```python
from build123d import *

# Parameters (mm, degrees)
BOSS_EXTRUDE1_DEPTH = 8.255
FILLET1_R           = 4.191
SKETCH2_R           = 2.07899
CUT_EXTRUDE1_DEPTH  = 81.896006892
FILLET2_R           = 4.191
SKETCH3_R           = 2.07899
CUT_EXTRUDE2_DEPTH  = 8.255


with BuildPart() as part:
    # Sketch1 → Boss-Extrude1 (new body)
    with BuildSketch(Plane(origin=(0, 0, 0), x_dir=(1, 0, 0), z_dir=(0, 1, 0))):
        Polygon((69.85, -7.99998), (69.85, -9.99998), (0, -9.99998), (0, -8.001), (9.99998, -8.001), (9.99998, -1.99898), (0, -1.99898), (0, 0), (69.85, 0), (69.85, -2), (79.84998, -2), (79.84998, -7.99998), align=None)
    extrude(amount=BOSS_EXTRUDE1_DEPTH)

    # Fillet1
    # the kernel refuses this fillet: 4.191 mm, written as the material it takes off along each edge
    with BuildSketch(Plane(origin=(0, 0, 12.47648), x_dir=(0, 1, 0), z_dir=(0, 0, -1)), Plane(origin=(0, 0, 20.47748), x_dir=(0, 1, 0), z_dir=(0, 0, -1))) as fillet1_piece_1:
        with BuildLine():
            CenterArc((FILLET1_R, FILLET1_R), FILLET1_R, 180, 90)
            Line((0, FILLET1_R), (0, 0))
            Line((0, 0), (FILLET1_R, 0))
        make_face()
    extrude(amount=22.95398, mode=Mode.SUBTRACT)
    with BuildSketch(Plane(origin=(0, 8.255, 12.47648), x_dir=(0, -1, 0), z_dir=(0, 0, -1)), Plane(origin=(0, 8.255, 20.47748), x_dir=(0, -1, 0), z_dir=(0, 0, -1))) as fillet1_piece_2:
        with BuildLine():
            CenterArc((FILLET1_R, -FILLET1_R), FILLET1_R, 90, 90)
            Line((0, -FILLET1_R), (0, 0))
            Line((0, 0), (FILLET1_R, 0))
        make_face()
    extrude(amount=22.95398, mode=Mode.SUBTRACT)

    # Sketch2 → Cut-Extrude1 (cut, through all)
    with BuildSketch(Plane.XY.offset(9.99998)):
        with Locations((2.587471088, 4.1275)):
            Circle(SKETCH2_R)
    extrude(amount=-CUT_EXTRUDE1_DEPTH, mode=Mode.SUBTRACT)

    # Fillet2
    # the kernel refuses this fillet: 4.191 mm, written as the material it takes off along each edge
    with BuildSketch(Plane(origin=(79.84998, 0, -8.4775), x_dir=(-1, 0, 0), z_dir=(0, 0, 1))) as fillet2_piece_1:
        with BuildLine():
            CenterArc((FILLET2_R, -FILLET2_R), FILLET2_R, 90, 90)
            Line((0, -FILLET2_R), (0, 0))
            Line((0, 0), (FILLET2_R, 0))
        make_face()
    extrude(amount=26.95498, mode=Mode.SUBTRACT)
    with BuildSketch(Plane(origin=(79.84998, 8.255, -8.4775), x_dir=(-1, 0, 0), z_dir=(0, 0, 1))) as fillet2_piece_2:
        with BuildLine():
            CenterArc((FILLET2_R, FILLET2_R), FILLET2_R, 180, 90)
            Line((0, FILLET2_R), (0, 0))
            Line((0, 0), (FILLET2_R, 0))
        make_face()
    extrude(amount=26.95498, mode=Mode.SUBTRACT)

    # Sketch3 → Cut-Extrude2 (cut)
    with BuildSketch(Plane.XY.offset(7.99998)):
        with Locations((75.65898, 4.191)):
            Circle(SKETCH3_R)
    extrude(amount=-CUT_EXTRUDE2_DEPTH, mode=Mode.SUBTRACT)


solid = part.part
```
Can you work these out from the model? Positions are in its coordinate system, mm. A direction names the side the tool comes from. Round coordinates to 2 decimals unless told otherwise and drop trailing zeros. Loops run counter-clockwise (first coordinate to the right, second up) from the corner with the lowest first, then second, coordinate; pieces in that order, holes last. Notation, with made-up numbers: M 52.25,80 L 89.25,80 A21 cw 89.25,94 Z; hole C -28.5,-33 d6. An arc over 180 degrees is marked long. Answer in a Markdown table with one row per item.
1. Thinking about a two-plate mould opening in X: for faces 6 (the face through (78.63, 7.02, 4.96)), 7 (the face through (1.2, 7, 9)), 8 (the face through (34, 4, 0)), 9 (the face through (4.57, 4.75, 1.01)), which applies, pulls with the +X half, pulls with the -X half, needs draft (parallel to the pull), parting line crosses it, or undercut?
Established:
| item | result |
|---|---|
| face 6 | pulls with the +X half |
| face 7 | pulls with the -X half |
| face 8 | needs draft |
| face 9 | undercut |
2. On a 3-axis mill with a long thin cutter (end or side, diameter ignored), from which of +Z, -Z, +X, -X, +Y, -Y can I reach the whole of each face in a straight line? I mean faces 1 (the face through (35, 4, 10)), 2 (the face through (69.85, 4, 9)), 3 (the face through (6, 4, 1.999)), 4 (the face through (73.67, 3.15, 2)), 5 (the face through (40, 8.255, 5)). Say none if no direction works.
Established:
| item | result |
|---|---|
| face 1 | +Z, +X, -X, +Y, -Y |
| face 2 | +Z, +X, +Y, -Y |
| face 3 | -X, +Y, -Y |
| face 4 | -Z, +X, +Y, -Y |
| face 5 | +Z, -Z, +X, -X, +Y |
3. If we section it at D-D, the plane y = 7.5: Please give me the cut outline in (x, z).
Established:
| item | result |
|---|---|
| outline | M 1.79,0 L 69.85,0 L 69.85,2 L 78.06,2 L 78.06,8 L 69.85,8 L 69.85,10 L 1.79,10 L 1.79,8 L 10,8 L 10,2 L 1.79,2 Z |
4. If we section it at C-C, the plane z = 4: Please give me the cut outline in (x, y) (1 decimal).
Established:
| item | result |
|---|---|
| outline | M 10,0 L 75.7,0 A4.2 ccw 79.8,4.1 A4.2 ccw 75.7,8.3 L 10,8.3 Z; hole C 75.7,4.2 d4.2 |
5. If we section it at A-A, the plane x = 5.5: Please give me the cut outline in (y, z) (3 decimals).
Established:
| item | result |
|---|---|
| outline | M 0,0 L 8.255,0 L 8.255,1.999 L 0,1.999 Z; M 0,8.001 L 8.255,8.001 L 8.255,10 L 0,10 Z |
6. If we section it at B-B, the plane y = 3: Please give me the cut outline in (x, z).
Established:
| item | result |
|---|---|
| outline | M 0.17,0 L 0.84,0 L 0.84,2 L 0.17,2 Z; M 0.17,8 L 0.84,8 L 0.84,10 L 0.17,10 Z; M 4.33,0 L 69.85,0 L 69.85,2 L 73.95,2 L 73.95,8 L 69.85,8 L 69.85,10 L 4.33,10 L 4.33,8 L 10,8 L 10,2 L 4.33,2 Z; M 77.36,2 L 79.68,2 L 79.68,8 L 77.36,8 Z |
7. Please list where these lines run through material, in increasing order: line 1 (Z direction, x = 6, y = 4.75); line 2 (X direction, y = 3.25, z = 8.25); line 3 (X direction, y = 3.75, z = 7.75). Write a range as from..to.
Established:
| item | result |
|---|---|
| line 1 | 0..2, 8..10 |
| line 2 | 0.11..0.7, 4.47..69.85 |
| line 3 | 10..73.63, 77.69..79.83 |
8. I'm going to push flat-ended pins straight in: pin 1 Ø1.5 at (y, z) = (1, 5) entering from -X; pin 2 Ø3 at (y, z) = (6, 5.5) entering from +X; pin 3 Ø0.6 at (y, z) = (4, 9.5) entering from +X. Where does each tip first touch, or does it pass through?
Established:
| item | result |
|---|---|
| pin 1 | x = 10 |
| pin 2 | x = 79.83 |
| pin 3 | x = 69.85 |
